```python
from build123d import *

# Parameters (mm, degrees)
CROQUIS1_R              = 12
SALIENTE_EXTRUIR1_DEPTH = 110
CROQUIS3_R              = 11
CORTAR_EXTRUIR1_DEPTH   = 110
CROQUIS4_R              = 15
SALIENTE_EXTRUIR3_DEPTH = 10
REDONDEO1_R             = 5
SALIENTE_EXTRUIR4_START = -10
CROQUIS5_R              = 15
SALIENTE_EXTRUIR4_DEPTH = 10
REDONDEO2_R             = 5
CORTAR_EXTRUIR2_START   = -100
CROQUIS7_R              = 11
CORTAR_EXTRUIR2_DEPTH   = 100
SALIENTE_EXTRUIR5_DEPTH = 0.75
MATRIZC1_COUNT          = 4


with BuildPart() as part:
    # Croquis1 → Saliente-Extruir1 (new body)
    with BuildSketch(Plane(origin=(0, 0, 0), x_dir=(0, 0, -1), z_dir=(1, 0, 0))):
        Circle(CROQUIS1_R)
    extrude(amount=SALIENTE_EXTRUIR1_DEPTH)

    # Croquis3 → Cortar-Extruir1 (cut)
    with BuildSketch(Plane(origin=(110, 0, 0), x_dir=(0, 0, -1), z_dir=(1, 0, 0))):
        Circle(CROQUIS3_R)
    extrude(amount=-CORTAR_EXTRUIR1_DEPTH, mode=Mode.SUBTRACT)

    # Croquis4 → Saliente-Extruir3 (add)
    with BuildSketch(Plane(origin=(110, 0, 0), x_dir=(0, 0, -1), z_dir=(1, 0, 0))):
        Circle(CROQUIS4_R)
    extrude(amount=-SALIENTE_EXTRUIR3_DEPTH)

    # Redondeo1
    # the kernel refuses this fillet: 5 mm, written as the material it takes off along each edge
    with BuildSketch(Plane(origin=(110, 0, 0), x_dir=(0, 0, -1), z_dir=(0, -1, 0))) as redondeo1_piece_1:
        with BuildLine():
            CenterArc((15 - REDONDEO1_R, -REDONDEO1_R), REDONDEO1_R, 0, 90)
            Line((15 - REDONDEO1_R, 0), (15 - REDONDEO1_R, REDONDEO1_R * 0.02))
            Line((15 - REDONDEO1_R, REDONDEO1_R * 0.02), (15 + REDONDEO1_R * 0.02, REDONDEO1_R * 0.02))
            Line((15 + REDONDEO1_R * 0.02, REDONDEO1_R * 0.02), (15 + REDONDEO1_R * 0.02, -REDONDEO1_R))
            Line((15 + REDONDEO1_R * 0.02, -REDONDEO1_R), (15, -REDONDEO1_R))
        make_face()
    revolve(axis=Axis((110, 0, 0), (1, 0, 0)), mode=Mode.SUBTRACT)
    with BuildSketch(Plane(origin=(100, 0, 0), x_dir=(0, 0, -1), z_dir=(0, -1, 0))) as redondeo1_piece_2:
        with BuildLine():
            CenterArc((10, 4.582575695), REDONDEO1_R, 293.578178478, 66.421821522)
            Line((15, 4.582575695), (15.1, 4.582575695))
            Line((15.1, 4.582575695), (15.1, 0))
            Line((15.1, 0), (15, -0.1))
            ThreePointArc((15, -0.1), (13.5, -0.1), (12.04, -0.091651514))
            Line((12.04, -0.091651514), (12, 0))
        make_face()
    revolve(axis=Axis((100, 0, 0), (1, 0, 0)), mode=Mode.SUBTRACT)

    # Croquis5 → Saliente-Extruir4 (add)
    with BuildSketch(Plane.ZY.offset(SALIENTE_EXTRUIR4_START)):
        with Locations(Location((0, 0, 0), (0, 0, 180))):
            Circle(CROQUIS5_R)
    extrude(amount=SALIENTE_EXTRUIR4_DEPTH)

    # Redondeo2
    # the kernel refuses this fillet: 5 mm, written as the material it takes off along each edge
    with BuildSketch(Plane(origin=(0, 0, 0), x_dir=(0, 0, -1), z_dir=(0, 1, 0))) as redondeo2_piece_1:
        with BuildLine():
            CenterArc((15 - REDONDEO2_R, -REDONDEO2_R), REDONDEO2_R, 0, 90)
            Line((15, -REDONDEO2_R), (15 + REDONDEO2_R * 0.02, -REDONDEO2_R))
            Line((15 + REDONDEO2_R * 0.02, -REDONDEO2_R), (15 + REDONDEO2_R * 0.02, REDONDEO2_R * 0.02))
            Line((15 + REDONDEO2_R * 0.02, REDONDEO2_R * 0.02), (15 - REDONDEO2_R, REDONDEO2_R * 0.02))
            Line((15 - REDONDEO2_R, REDONDEO2_R * 0.02), (15 - REDONDEO2_R, 0))
        make_face()
    revolve(axis=Axis((0, 0, 0), (-1, 0, 0)), mode=Mode.SUBTRACT)
    with BuildSketch(Plane(origin=(10, 0, 0), x_dir=(0, 0, -1), z_dir=(0, 1, 0))) as redondeo2_piece_2:
        with BuildLine():
            CenterArc((10, 4.582575695), REDONDEO2_R, 293.578178478, 66.421821522)
            Line((12, 0), (12.04, -0.091651514))
            ThreePointArc((12.04, -0.091651514), (13.5, -0.1), (15, -0.1))
            Line((15, -0.1), (15.1, 0))
            Line((15.1, 0), (15.1, 4.582575695))
            Line((15.1, 4.582575695), (15, 4.582575695))
        make_face()
    revolve(axis=Axis((10, 0, 0), (-1, 0, 0)), mode=Mode.SUBTRACT)

    # Croquis7 → Cortar-Extruir2 (cut)
    with BuildSketch(Plane.ZY.offset(CORTAR_EXTRUIR2_START)):
        with Locations(Location((0, 0, 0), (0, 0, 180))):
            Circle(CROQUIS7_R)
    extrude(amount=CORTAR_EXTRUIR2_DEPTH, mode=Mode.SUBTRACT)

    # Croquis9 → Saliente-Extruir5 (add, symmetric)
    with BuildSketch(Plane.XY.offset(11.985010852)):
        Polygon((18.375194252, 0), (27.66376902, 5.462495064), (36.886888429, -0.109806246), (27.598313662, -5.57230131), align=None)
        Polygon((45.375194252, 0), (54.66376902, 5.462495064), (63.886888429, -0.109806246), (54.598313662, -5.57230131), align=None)
        Polygon((72.375194252, 0), (81.66376902, 5.462495064), (90.886888429, -0.109806246), (81.598313662, -5.57230131), align=None)
    saliente_extruir5 = extrude(amount=SALIENTE_EXTRUIR5_DEPTH, both=True)

    # MatrizC1: Saliente-Extruir5 ×4 about axis
    matrizc1_axis = Axis((0, 0, 0), (1, 0, 0))
    for i in range(1, MATRIZC1_COUNT):
        add(saliente_extruir5.rotate(matrizc1_axis, i * 360 / MATRIZC1_COUNT))


solid = part.part
```
The listing builds one solid part. Answer for the finished solid, in the listing's coordinates (mm). A direction names the side the tool comes from. Coordinates: 2 decimals unless noted, no trailing zeros. Write each loop counter-clockwise with the first axis right and the second up, starting at its lowest first coordinate (ties: lowest second). Pieces come first, ordered by that corner, then holes. Notation, with made-up numbers: (31.5, 5.25) - (58.5, 5.25) arc R17 cw to (58.5, 17.25) - close; hole circle Ø4 at (-22, 71.5). An arc over 180 degrees is marked (long way). Return JSON: item names as keys, results as strings. Group by question number.
1. Which of the six approach directions +Z, -Z, +X, -X, +Y, -Y give full straight-line access (tool end or side, diameter ignored) to faces 1 (the flat face through (55, 0, 12.735)), 2 (the flat face through (78.076, 12.162, 3.444)), 3 (the flat face through (78.076, -12.162, -3.444)), 4 (the flat face through (77.99, -12.16, 3.3)), 5 (the flat face through (82, 0, -12.735))?
2. Determine the mould class of faces 6 (the flat face through (55, 12.735, 0)), 7 (the cylindrical face through (5.21, -12.65, -8.06)) for opening direction X: released by +X, released by -X, zero draft, split by the parting line, or undercut.
3. Given pin 1 (2 mm diameter, centred on x = 82, z = 9, fed in from -Y); pin 2 (3.5 mm diameter, centred on x = 51, z = -2.5, fed in from +Y) (3 decimals); pin 3 (1 mm diameter, centred on x = 27.5, y = -5, fed in from +Z) (3 decimals); pin 4 (8 mm diameter, centred on y = 8.5, z = -8.5, fed in from +X), each flat-ended and moving along its own axis, determine where each tip first touches the part or whether it passes through.
4. Straight lines are drawn through the part: L1, parallel to Y at x = 22, z = 0; L2, parallel to X at y = 5.5, z = -12.5; L3, parallel to Y at x = 37.5, z = 0. For each, find the intervals that lie inside material, in ascending order.
5. A cutting plane is placed at A-A, the plane x = 86. Determine the outline of the cut face in (y, z), plus the area to 3 significant figures.
Ans:
{
 "1": {"face 1": "+Z, +Y, -Y", "face 2": "+Z, +Y", "face 3": "-Z, -Y", "face 4": "+Z, -Y", "face 5": "-Z, +Y, -Y"},
 "2": {"face 6": "undercut", "face 7": "zero draft"},
 "3": {"pin 1": "y = -8.94", "pin 2": "y = 12.735", "pin 3": "z = 12.735", "pin 4": "x = 110"},
 "4": {"L1": "-12.74 to -11, 11 to 12.74", "L2": "1.59 to 8.83, 27.48 to 27.72, 54.48 to 54.72, 81.48 to 81.72, 101.17 to 108.41", "L3": "-12 to -11, 11 to 12"},
 "5": {"outline": "(-12.74, -2.98) - (-11.62, -2.98) arc R12 ccw to (-2.84, -11.66) - (-2.84, -12.74) - (2.98, -12.74) - (2.98, -11.62) arc R12 ccw to (11.66, -2.84) - (12.74, -2.84) - (12.74, 2.98) - (11.62, 2.98) arc R12 ccw to (2.84, 11.66) - (2.84, 12.74) - (-2.98, 12.74) - (-2.98, 11.62) arc R12 ccw to (-11.66, 2.84) - (-12.74, 2.84) - close; hole circle Ø22 at (0, 0)", "area": "92.2 mm²"}
}
